Design review of the part built by this model. Coordinates are the model's own, in mm. A direction names the side the tool comes from. Coordinates: 2 decimals unless noted, no trailing zeros. Loops run counter-clockwise (first coordinate to the right, second up) from the corner with the lowest first, then second, coordinate; pieces in that order, holes last. Notation, with made-up numbers: M 14.25,-8.75 L 58.25,-8.75 A25 cw 58.25,4.25 Z; hole C -25.75,-26 d10. An arc over 180 degrees is marked long. Put each result on its own line as item: value. Start each with the question number.
(1) The part is to be moulded in two halves that separate along X. For faces 1 (the cylindrical face through (-2.06, 42.87, 2.46)), 2 (the flat face through (160, 20, 2)), 3 (the flat face through (-2, 48, 5)), say which applies: +X half, -X half, draft (parallel to the pull), parting line (faces both ways), or undercut.
(2) Clearance check with flat-ended pins moving along their axes: pin 1 (1 mm diameter, centred on y = 54, z = 2.5, fed in from +X); pin 2 (5 mm diameter, centred on x = -150, y = 10, fed in from -Z); pin 3 (3.5 mm diameter, centred on x = 20, y = 70, fed in from -Z). State where each tip first meets the part, or that it passes through.
(3) For faces 4 (the flat face through (-149, 0, 2)), 5 (the flat face through (149, 40, 2)), 6 (the flat face through (-148, 40, 2)), list the 3-axis set-ups (+Z, -Z, +X, -X, +Y, -Y) from which the entire face can be reached by the end or side of a thin tool; tool diameter is ignored.
(4) Take a section at B-B, the plane x = 10. Give the boundary of the cut face in (y, z).
(5) Take a section at A-A, the plane z = 1.2. Count the separate pieces of the cut face and the enclosed holes in it, then the cut area to 3 significant figures.
(6) For probe 1 along Y at (x, z) = (-150, 3.05); probe 2 along Y at (x, z) = (20, 3.9); probe 3 along X at (y, z) = (5, 1.25), list the stretches that pass through material, from the lowest coordinate up. Write a range as [from, to].
(7) Take a section at C-C, the plane x = 93.5. Give the boundary of the cut face in (y, z), then the cut area to 3 significant figures.
```python
from build123d import *

# Parameters (mm, degrees)
ESQUISSE1_R        = 2
BOSS_EXTRU_1_DEPTH = 5
CONG_1_R           = 4


with BuildPart() as part:
    # Esquisse1 → Boss.-Extru.1 (new body)
    with BuildSketch(Plane.XY):
        with BuildLine():
            Line((160, 0), (160, 40))
            Line((160, 40), (140, 40))
            ThreePointArc((140, 40), (0, 76.901234754), (-140, 40))
            Line((-140, 40), (-160, 40))
            Line((-160, 40), (-160, 0))
            Line((-160, 0), (-140, 0))
            ThreePointArc((-140, 0), (0, 42.876848228), (140, 0))
            Line((140, 0), (160, 0))
        make_face()
        with Locations((20, 70)):
            Circle(ESQUISSE1_R, mode=Mode.SUBTRACT)
        with Locations((20, 50)):
            Circle(ESQUISSE1_R, mode=Mode.SUBTRACT)
        with Locations(Location((-20, 50, 0), (0, 0, 180))):
            Circle(ESQUISSE1_R, mode=Mode.SUBTRACT)
        with Locations(Location((-20, 70, 0), (0, 0, 180))):
            Circle(ESQUISSE1_R, mode=Mode.SUBTRACT)
        with Locations((150, 30)):
            Circle(ESQUISSE1_R, mode=Mode.SUBTRACT)
        with Locations((150, 10)):
            Circle(ESQUISSE1_R, mode=Mode.SUBTRACT)
        with Locations(Location((-150, 10, 0), (0, 0, 180))):
            Circle(ESQUISSE1_R, mode=Mode.SUBTRACT)
        with Locations(Location((-150, 30, 0), (0, 0, 180))):
            Circle(ESQUISSE1_R, mode=Mode.SUBTRACT)
    extrude(amount=BOSS_EXTRU_1_DEPTH)

    # Congé1
    cong_1_edges = [part.edges().sort_by_distance(p)[0] for p in [
        (-140, 0, 2.5),
        (-160, 0, 2.5),
        (-160, 40, 2.5),
        (-140, 40, 2.5),
        (140, 40, 2.5),
        (160, 40, 2.5),
        (160, 0, 2.5),
        (140, 0, 2.5),
    ]]
    fillet(cong_1_edges, radius=CONG_1_R)


solid = part.part
```
Computed values:
1. face 1: undercut
1. face 2: +X half
1. face 3: draft
2. pin 1: stops at x = 112.9
2. pin 2: stops at z = 0
2. pin 3: passes through
3. face 4: +Z, -Z, +X, -X, -Y
3. face 5: +Z, -Z, +X, +Y
3. face 6: +Z, -Z, -X, +Y
4. outline: M 42.68,0 L 76.73,0 L 76.73,5 L 42.68,5 Z
5. separate pieces: 1
5. enclosed holes: 8
5. area: 11,500 mm^2
6. probe 1: y = [0, 8], [12, 28], [32, 40]
6. probe 2: y = [42.08, 48], [52, 68], [72, 76.2]
6. probe 3: x = [-160, -132.3], [132.3, 160]
7. outline: M 24.73,0 L 61.07,0 L 61.07,5 L 24.73,5 Z
7. area: 182 mm^2
